```python
from build123d import *

# Parameters (mm, degrees)
BOSS_EXTRUDE1_DEPTH = 25
CUT_EXTRUDE1_DEPTH  = 1


with BuildPart() as part:
    # Sketch1 → Boss-Extrude1 (new body)
    with BuildSketch(Plane(origin=(0, 0, 0), x_dir=(1, 0, 0), z_dir=(0, 1, 0))):
        Polygon((0, 0), (0, 100), (100, 100), (100, -100), (-200, -100), (-200, 0), align=None)
    extrude(amount=BOSS_EXTRUDE1_DEPTH)

    # Sketch2 → Cut-Extrude1 (cut)
    with BuildSketch(Plane(origin=(0, 25, 0), x_dir=(1, 0, 0), z_dir=(0, 1, 0))):
        Polygon((150.414178645, 73.750443427), (-91.067277928, 9.045682152), (-91.843735063, 11.943459631), (149.637721509, 76.648220906), align=None)
    extrude(amount=-CUT_EXTRUDE1_DEPTH, mode=Mode.SUBTRACT)


solid = part.part
```
Read the model definition and answer for the solid it produces. Units are mm, in the model's axes. A direction names the side the tool comes from. Give positions to 0.01 mm unless a question says otherwise; leave off trailing zeros. Order: outer loops, then holes, each group sorted by start corner. A loop starts at its lowest first (then second) coordinate and runs counter-clockwise, first axis right, second up.
(1) For a pull along Z with two mould halves and no side action, classify faces 4 (the flat face through (-48, 25, 37)), 5 (the flat face through (-101, 12, 0)), 6 (the flat face through (49.3, 24.507, -49.763)) as released by +Z, released by -Z, zero draft, split by the parting line, or undercut.
(2) Find section B-B (x = -156.5). Give the vertices of the cut face in (y, z), plus the area to 3 significant figures.
(3) For faces 1 (the flat face through (50, 24, -48)), 2 (the flat face through (0, 12, -49)), 3 (the flat face through (-15, 0, 21)), determine the directions among +Z, -Z, +X, -X, +Y, -Y from which every point of the face is accessible in a straight line to the end or side of a thin tool.
(4) Find section A-A (y = 9.5). Give the vertices of the cut face in (x, z), plus the area to 3 significant figures.
(5) A straight line is drawn through the part: L1, parallel to Z at x = -96.5, y = 21.25. Find the intervals that lie inside material, in ascending order.
(6) Given pin 1 (6 mm diameter, centred on y = 8.5, z = -44.5, fed in from -X); pin 2 (3 mm diameter, centred on x = -65.5, y = 15.5, fed in from -Z), each flat-ended and moving along its own axis, determine where each tip first touches the part or whether it passes through.
Result sheet:
1. face 4: zero draft
1. face 5: released by -Z
1. face 6: undercut
2. outline: (0, 0) - (25, 0) - (25, 100) - (0, 100) - close
2. area: 2,500 mm2
3. face 1: +Y
3. face 2: -Z, -X, +Y, -Y
3. face 3: +Z, -Z, +X, -X, -Y
4. outline: (-200, 0) - (0, 0) - (0, -100) - (100, -100) - (100, 100) - (-200, 100) - close
4. area: 40,000 mm2
5. L1: z = 0 to 100
6. pin 1: stops at x = 0
6. pin 2: stops at z = 0
